```python
from build123d import *

# Parameters (mm, degrees)
SKETCH_2_W          = 85
SKETCH_2_H          = 85
SKETCH_2_W_2        = 75
SKETCH_2_H_2        = 75
EXTRUDE_1_DEPTH     = 70
SKETCH_3_R          = 21.1
CUT_EXTRUDE_1_DEPTH = 10
SKETCH_4_R          = 1.25
CUT_EXTRUDE_2_DEPTH = 10
FILLET_1_R          = 5
FILLET_2_R          = 10
SKETCH_5_W          = 97.414855886
SKETCH_5_H          = 125.778371442
CUT_EXTRUDE_3_DEPTH = 8
SKETCH_6_R          = 5
CUT_EXTRUDE_4_DEPTH = 10
SKETCH_13_R         = 7.5
SKETCH_13_R_2       = 2.5
CUT_EXTRUDE_7_DEPTH = 31
SKETCH_15_W         = 20
SKETCH_15_H         = 16
CUT_EXTRUDE_8_DEPTH = 12
CUT_EXTRUDE_9_DEPTH = 12


with BuildPart() as part:
    # Sketch 2 → Extrude 1 (new body)
    with BuildSketch(Plane(origin=(0, 0, 0), x_dir=(0, 0, -1), z_dir=(1, 0, 0))):
        Rectangle(SKETCH_2_W, SKETCH_2_H)
        Rectangle(SKETCH_2_W_2, SKETCH_2_H_2, mode=Mode.SUBTRACT)
    extrude(amount=EXTRUDE_1_DEPTH)

    # Sketch 3 → Cut-Extrude 1 (cut)
    with BuildSketch(Plane.XY.offset(-37.5)):
        with Locations((35, 8.5)):
            Circle(SKETCH_3_R)
    cut_extrude_1 = extrude(amount=-CUT_EXTRUDE_1_DEPTH, mode=Mode.SUBTRACT)

    # Sketch 4 → Cut-Extrude 2 (cut)
    with BuildSketch(Plane.XY.offset(-37.5)):
        with Locations((14.5, 20.335680518)):
            Circle(SKETCH_4_R)
        with Locations((35, -15.171361037)):
            Circle(SKETCH_4_R)
        with Locations((55.5, 20.335680518)):
            Circle(SKETCH_4_R)
    cut_extrude_2 = extrude(amount=-CUT_EXTRUDE_2_DEPTH, mode=Mode.SUBTRACT)

    # Mirror 1: Cut-Extrude 1, Cut-Extrude 2 across plane
    add(cut_extrude_1.mirror(Plane(origin=(0, 0, 0), x_dir=(0, 0.707106781, 0.707106781), z_dir=(0, 0.707106781, -0.707106781))), mode=Mode.SUBTRACT)
    add(cut_extrude_2.mirror(Plane(origin=(0, 0, 0), x_dir=(0, 0.707106781, 0.707106781), z_dir=(0, 0.707106781, -0.707106781))), mode=Mode.SUBTRACT)

    # Fillet 1
    fillet_1_edges = [part.edges().sort_by_distance(p)[0] for p in [
        (35, -37.5, -37.5),
        (35, 37.5, -37.5),
        (35, 37.5, 37.5),
        (35, -37.5, 37.5),
    ]]
    fillet(fillet_1_edges, radius=FILLET_1_R)

    # Fillet 2
    fillet_2_edges = [part.edges().sort_by_distance(p)[0] for p in [
        (35, 42.5, 42.5),
        (35, 42.5, -42.5),
        (35, -42.5, -42.5),
        (35, -42.5, 42.5),
    ]]
    fillet(fillet_2_edges, radius=FILLET_2_R)

    # Sketch 5 → Cut-Extrude 3 (cut)
    with BuildSketch(Plane.ZY):
        Rectangle(SKETCH_5_W, SKETCH_5_H)
    extrude(amount=-CUT_EXTRUDE_3_DEPTH, mode=Mode.SUBTRACT)

    # Sketch 6 → Cut-Extrude 4 (cut)
    with BuildSketch(Plane(origin=(0, 42.5, 0), x_dir=(1, 0, 0), z_dir=(0, 1, 0))):
        with Locations((35, 18.85)):
            Circle(SKETCH_6_R)
    cut_extrude_4 = extrude(amount=-CUT_EXTRUDE_4_DEPTH, mode=Mode.SUBTRACT)

    # Mirror 2: Cut-Extrude 4 across plane
    add(cut_extrude_4.mirror(Plane(origin=(0, 0, 0), x_dir=(0, 0.707106781, 0.707106781), z_dir=(0, 0.707106781, -0.707106781))), mode=Mode.SUBTRACT)

    # Sketch 13 → Cut-Extrude 7 (cut)
    with BuildSketch(Plane(origin=(0, 42.5, 0), x_dir=(1, 0, 0), z_dir=(0, 1, 0))):
        with Locations((35, -8.5)):
            Circle(SKETCH_13_R)
        with Locations((55.5, -20.335680518)):
            Circle(SKETCH_13_R_2)
        with Locations((14.5, -20.335680518)):
            Circle(SKETCH_13_R_2)
    cut_extrude_7 = extrude(amount=-CUT_EXTRUDE_7_DEPTH, mode=Mode.SUBTRACT)

    # Mirror 5: Cut-Extrude 7 across plane
    add(cut_extrude_7.mirror(Plane(origin=(0, 0, 0), x_dir=(0, 0.707106781, 0.707106781), z_dir=(0, 0.707106781, -0.707106781))), mode=Mode.SUBTRACT)

    # Sketch 15 → Cut-Extrude 8 (cut)
    with BuildSketch(Plane.XY.offset(-37.5)):
        with Locations((60, -29.5)):
            Rectangle(SKETCH_15_W, SKETCH_15_H)
    extrude(amount=CUT_EXTRUDE_8_DEPTH, mode=Mode.SUBTRACT)

    # Sketch 16 → Cut-Extrude 9 (cut)
    with BuildSketch(Plane.XY.offset(-37.5)):
        with BuildLine():
            Line((65, -17.990833729), (70, -17.990833729))
            ThreePointArc((70, -17.990833729), (72, -19.990833729), (70, -21.990833729))
            Line((70, -21.990833729), (65, -21.990833729))
            ThreePointArc((65, -21.990833729), (63, -19.990833729), (65, -17.990833729))
        make_face()
    extrude(amount=-CUT_EXTRUDE_9_DEPTH, mode=Mode.SUBTRACT)


solid = part.part
```
The model under review builds one solid part; all positions refer to its coordinate system, in mm. A direction names the side the tool comes from. Round coordinates to 2 decimals unless told otherwise and drop trailing zeros. Write each loop counter-clockwise with the first axis right and the second up, starting at its lowest first coordinate (ties: lowest second). Pieces come first, ordered by that corner, then holes.
(1) We need section C-C on z = -18.85. Give the boundary of the cut face in (x, y).
(2) Mouldability with a two-part tool opening along Z and no side actions: class faces 1 (the cylindrical face through (39.43, 36.07, 36)), 2 (the flat face through (39, 0, 37.5)), 3 (the flat face through (67, -17.991, -40)), 4 (the cylindrical face through (39.43, 39.49, 39.65)) as +Z half, -Z half, draft (parallel to the pull), parting line (faces both ways), or undercut.
(3) Machinability: for faces 5 (the flat face through (39, 37.5, 0)), 6 (the cylindrical face through (57.885, 40.035, 19.585)), 7 (the flat face through (68, -21.991, -40)), 8 (the cylindrical face through (56.8, 18.2, 40)), which of the approach directions +Z, -Z, +X, -X, +Y, -Y give a long, thin tool a straight path to every point of the face, cutting with its end or side? Answer none if there is none.
(4) Wall thickness on L1, parallel to Z at x = 30.5, y = -14.5; L2, parallel to Y at x = 27, z = -9: over which ranges is each line inside the solid? List them lowest first.
(5) We need section D-D on y = -6. Give the boundary of the cut face in (x, z).
(6) We need section A-A on y = 8.5. Give the boundary of the cut face in (x, z).
(7) Insertion check: pin 1 (2 mm diameter, centred on x = 14.5, y = 20.34, fed in from +Z); pin 2 (4 mm diameter, centred on x = 55.5, y = 20.34, fed in from +Z); pin 3 (1.5 mm diameter, centred on x = 68.5, z = -41, fed in from -Y); pin 4 (4 mm diameter, centred on y = -34.5, z = -35, fed in from +X). Each pin has a flat end and moves straight along its axis. Give the tip position at first contact, or say it passes through.
Findings below:
1. outline: (8, -42.5) - (70, -42.5) - (70, -37.5) - (8, -37.5) - close; (8, 37.5) - (30, 37.5) - (30, 42.5) - (8, 42.5) - close; (40, 37.5) - (70, 37.5) - (70, 42.5) - (40, 42.5) - close
2. face 1: undercut
2. face 2: undercut
2. face 3: draft
2. face 4: +Z half
3. face 5: +X, -X
3. face 6: +Y
3. face 7: -Z, +X
3. face 8: +Z
4. L1: z = -42.5 to -37.5, 37.5 to 42.5
4. L2: y = 37.5 to 42.5
5. outline: (8, -42.5) - (19.67, -42.5) - (19.67, -37.5) - (8, -37.5) - close; (8, 37.5) - (70, 37.5) - (70, 42.5) - (8, 42.5) - close; (50.33, -42.5) - (70, -42.5) - (70, -37.5) - (50.33, -37.5) - close
6. outline: (8, -42.5) - (13.9, -42.5) - (13.9, -37.5) - (8, -37.5) - close; (8, 37.5) - (27.5, 37.5) - (27.5, 42.5) - (8, 42.5) - close; (42.5, 37.5) - (70, 37.5) - (70, 42.5) - (42.5, 42.5) - close; (56.1, -42.5) - (70, -42.5) - (70, -37.5) - (56.1, -37.5) - close
7. pin 1: passes through
7. pin 2: stops at z = -37.5
7. pin 3: stops at y = -38.82
7. pin 4: stops at x = 50
